The listing builds one solid part. Answer for the finished solid, in the listing's coordinates (mm). Face numbers are marked on the shaded views. A direction names the side the tool comes from. Give positions to 0.01 mm unless a question says otherwise; leave off trailing zeros. Order: outer loops, then holes, each group sorted by start corner. A loop starts at its lowest first (then second) coordinate and runs counter-clockwise, first axis right, second up. Notation, with made-up numbers: (27.5, 5) - (76.5, 5) arc R26 cw to (76.5, 25) - close; hole circle Ø5 at (13, -4.5). An arc over 180 degrees is marked (long way). Answer in a Markdown table with one row per item.
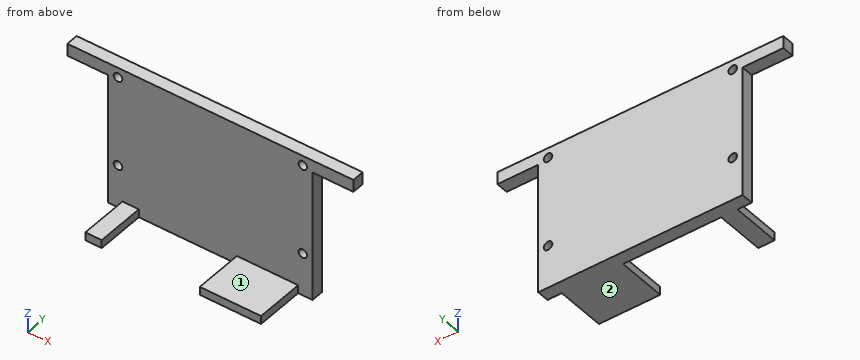
from build123d import *

# Parameters (mm, degrees)
BOSS_EXTRUDE1_DEPTH = 3
SKETCH2_R           = 1.05
CUT_EXTRUDE1_DEPTH  = 3
SKETCH3_R           = 1.05
CUT_EXTRUDE2_DEPTH  = 3
SKETCH4_W           = 15
SKETCH4_H           = 2
SKETCH4_W_2         = 4
BOSS_EXTRUDE2_DEPTH = 12


with BuildPart() as part:
    # Sketch1 → Boss-Extrude1 (new body)
    with BuildSketch(Plane(origin=(0, 0, 0), x_dir=(1, 0, 0), z_dir=(0, 1, 0))):
        Polygon((-26.238881315, 17.558528428), (23.761118685, 17.558528428), (23.761118685, -14.441471572), (33.761118685, -14.441471572), (33.761118685, -17.441471572), (23.761118685, -17.441471572), (-26.238881315, -17.441471572), (-36.238881315, -17.441471572), (-36.238881315, -14.441471572), (-26.238881315, -14.441471572), align=None)
    extrude(amount=BOSS_EXTRUDE1_DEPTH)

    # Sketch2 → Cut-Extrude1 (cut)
    with BuildSketch(Plane(origin=(0, 3, 0), x_dir=(1, 0, 0), z_dir=(0, 1, 0))):
        with Locations(Location((-23.838881315, -15.041471572, 0), (0, 0, 270))):
            Circle(SKETCH2_R)
        with Locations(Location((21.361118685, -15.041471572, 0), (0, 0, 270))):
            Circle(SKETCH2_R)
    extrude(amount=-CUT_EXTRUDE1_DEPTH, mode=Mode.SUBTRACT)

    # Sketch3 → Cut-Extrude2 (cut)
    with BuildSketch(Plane(origin=(0, 3, 0), x_dir=(1, 0, 0), z_dir=(0, 1, 0))):
        with Locations(Location((-23.838881315, 7.058528428, 0), (0, 0, 270))):
            Circle(SKETCH3_R)
        with Locations(Location((21.361118685, 7.058528428, 0), (0, 0, 270))):
            Circle(SKETCH3_R)
    extrude(amount=-CUT_EXTRUDE2_DEPTH, mode=Mode.SUBTRACT)

    # Sketch4 → Boss-Extrude2 (add)
    with BuildSketch(Plane.XZ):
        with Locations((12.761118685, -16.558528428)):
            Rectangle(SKETCH4_W, SKETCH4_H)
        with Locations((-20.738881315, -16.558528428)):
            Rectangle(SKETCH4_W_2, SKETCH4_H)
    extrude(amount=BOSS_EXTRUDE2_DEPTH)


solid = part.part
Item 1: Find section B-B on x = 6. Write down the section's boundary in (y, z), then the cut area to 3 significant figures.
Answer block:
| item | result |
|---|---|
| outline | (-12, -17.56) - (3, -17.56) - (3, 17.44) - (0, 17.44) - (0, -15.56) - (-12, -15.56) - close |
| area | 129 mm² |
Item 2: Each of these flat-tipped pins is pushed along its axis until it touches: P1, Ø1, axis at x = 17.5, y = -4.5, coming from the +Z side; P2, Ø1.3, axis at x = -23.84, z = 15.04, coming from the +Y side; P3, Ø1.5, axis at y = 1.5, z = -5.5, coming from the -X side; P4, Ø2, axis at y = -4.5, z = -16.5, coming from the +X side. Where does it stop, or does it pass through?
Answer block:
| item | result |
|---|---|
| P1 | z = -15.56 |
| P2 | through |
| P3 | x = -26.24 |
| P4 | x = 20.26 |
Item 3: Find section A-A on y = -7. Write down the section's boundary in (x, z).
Answer block:
| item | result |
|---|---|
| outline | (-22.74, -17.56) - (-18.74, -17.56) - (-18.74, -15.56) - (-22.74, -15.56) - close; (5.26, -17.56) - (20.26, -17.56) - (20.26, -15.56) - (5.26, -15.56) - close |
Item 4: Which of the six approach directions +Z, -Z, +X, -X, +Y, -Y give full straight-line access (tool end or side, diameter ignored) to the marked faces 1 and 2?
Answer block:
| item | result |
|---|---|
| face 1 | +Z, +X, -X, -Y |
| face 2 | -Z, +X, -X, +Y, -Y |
Item 5: Consider line 1 (Z direction, x = 16, y = -4); line 2 (Z direction, x = 28.5, y = 0.75); line 3 (X direction, y = 1.5, z = 10). Determine where each line is inside the solid, lowest interval first.
Answer block:
| item | result |
|---|---|
| line 1 | -17.56 to -15.56 |
| line 2 | 14.44 to 17.44 |
| line 3 | -26.24 to 23.76 |
Item 6: Find section C-C on y = 1. Write down the section's boundary in (x, z), then the cut area to 3 significant figures.
Answer block:
| item | result |
|---|---|
| outline | (-36.24, 14.44) - (-26.24, 14.44) - (-26.24, -17.56) - (23.76, -17.56) - (23.76, 14.44) - (33.76, 14.44) - (33.76, 17.44) - (-36.24, 17.44) - close; hole circle Ø2.1 at (-23.84, -7.06); hole circle Ø2.1 at (-23.84, 15.04); hole circle Ø2.1 at (21.36, -7.06); hole circle Ø2.1 at (21.36, 15.04) |
| area | 1,800 mm² |
Item 7: Find section D-D on z = 10.5. Write down the section's boundary in (x, y).
Answer block:
| item | result |
|---|---|
| outline | (-26.24, 0) - (23.76, 0) - (23.76, 3) - (-26.24, 3) - close |
